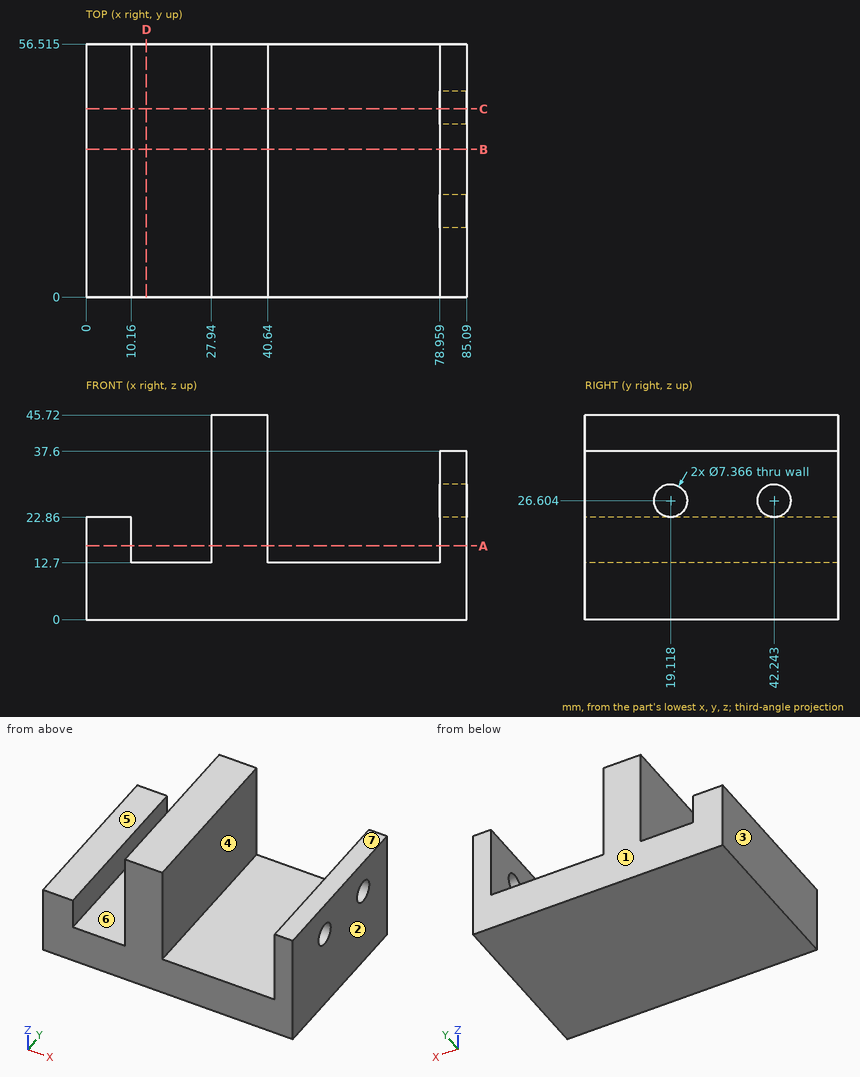
The drawing under review shows one solid part. Ordinate dimensions are in mm from its lowest x, y, z. A direction names the side the tool comes from. Round coordinates to 2 decimals unless told otherwise and drop trailing zeros. Write each loop counter-clockwise with the first axis right and the second up, starting at its lowest first coordinate (ties: lowest second). Pieces come first, ordered by that corner, then holes. Notation, with made-up numbers: (42.25, 68.5) - (97.25, 68.5) arc R26 ccw to (97.25, 87.5) - close; hole circle Ø11 at (-35.5, 5.25). An arc over 180 degrees is marked (long way). One line per question, with ' | ' between items.
Item 1: For P1, Ø9, axis at x = 19.5, y = 18, coming from the +Z side; P2, Ø8, axis at x = 3.5, y = 26, coming from the +Z side; P3, Ø3, axis at x = 43.5, z = 18, coming from the -Y side; P4, Ø4.5, axis at y = 19.12, z = 26.6, coming from the +X side, all flat-tipped, find the tip position at first contact; note any pin that passes through.
Resolved:
P1: stops at z = 12.7 | P2: stops at z = 22.86 | P3: passes through | P4: stops at x = 40.64
Item 2: To check wall thickness, follow probe 1 along X at (y, z) = (29.5, 22); probe 2 along Z at (x, y) = (47.5, 52.5); probe 3 along X at (y, z) = (52.5, 43). State the ranges of each line that lie inside material, in increasing order.
Resolved:
probe 1: x = 0 to 10.16, 27.94 to 40.64, 78.96 to 85.09 | probe 2: z = 0 to 12.7 | probe 3: x = 27.94 to 40.64
Item 3: Add section A-A, the plane z = 16.5. Give the boundary of the cut face in (x, y) (1 decimal), then the cut area to 3 significant figures.
Resolved:
outline: (0, 0) - (10.2, 0) - (10.2, 56.5) - (0, 56.5) - close; (27.9, 0) - (40.6, 0) - (40.6, 56.5) - (27.9, 56.5) - close; (79, 0) - (85.1, 0) - (85.1, 56.5) - (79, 56.5) - close | area: 1,640 mm2
Item 4: Add section B-B, the plane y = 33. Give the boundary of the cut face in (x, z).
Resolved:
outline: (0, 0) - (85.09, 0) - (85.09, 37.6) - (78.96, 37.6) - (78.96, 12.7) - (40.64, 12.7) - (40.64, 45.72) - (27.94, 45.72) - (27.94, 12.7) - (10.16, 12.7) - (10.16, 22.86) - (0, 22.86) - close
Item 5: Add section C-C, the plane y = 42. Give the boundary of the cut face in (x, z).
Resolved:
outline: (0, 0) - (85.09, 0) - (85.09, 22.93) - (78.96, 22.93) - (78.96, 12.7) - (40.64, 12.7) - (40.64, 45.72) - (27.94, 45.72) - (27.94, 12.7) - (10.16, 12.7) - (10.16, 22.86) - (0, 22.86) - close; (78.96, 30.28) - (85.09, 30.28) - (85.09, 37.6) - (78.96, 37.6) - close
Item 6: Add section D-D, the plane x = 13.5. Give the boundary of the cut face in (y, z) (1 decimal), then the cut area to 3 significant figures.
Resolved:
outline: (0, 0) - (56.5, 0) - (56.5, 12.7) - (0, 12.7) - close | area: 718 mm2
Item 7: The part is to be moulded in two halves that separate along X. For the marked faces 1, 2, 3 and 4, say which applies: pulls with the +X half, pulls with the -X half, needs draft (parallel to the pull), parting line crosses it, or undercut.
Resolved:
face 1: needs draft | face 2: pulls with the +X half | face 3: pulls with the -X half | face 4: undercut
Item 8: For the marked faces 5, 6 and 7, list the 3-axis set-ups (+Z, -Z, +X, -X, +Y, -Y) from which the entire face can be reached by the end or side of a thin tool; tool diameter is ignored.
Resolved:
face 5: +Z, -X, +Y, -Y | face 6: +Z, +Y, -Y | face 7: +Z, +X, +Y, -Y
